The model under review builds one solid part; all positions refer to its coordinate system, in mm. Coordinates: 2 decimals unless noted, no trailing zeros. Loops run counter-clockwise (first coordinate to the right, second up) from the corner with the lowest first, then second, coordinate; pieces in that order, holes last. Notation, with made-up numbers: M 56,-20 L 82,-20 A29 ccw 82,4 Z; hole C 27.5,53 d3. An arc over 180 degrees is marked long. Write item = value, one per line. Start each with the question number.
Q1. We need section A-A on y = -17. Give the boundary of the cut face in (x, z), and give its area (3 significant figures).
Q2. We need section B-B on z = 1.65. Give the boundary of the cut face in (x, y).
Q3. Wall thickness on probe 1 along X at (y, z) = (-13, 4.15); probe 2 along Y at (x, z) = (139, 0.3); probe 3 along X at (y, z) = (6.5, 2.55): over which ranges is each line inside the solid? List them lowest first.
Q4. Clearance check with flat-ended pins moving along their axes: pin 1 Ø2.5 at (x, z) = (-83, 3.5) entering from -Y; pin 2 Ø1.5 at (y, z) = (13.5, 3.5) entering from -X; pin 3 Ø2.5 at (y, z) = (18, 1.5) entering from +X. State where each tip first meets the part, or that it passes through.
Q5. We need section C-C on x = 144.5. Give the boundary of the cut face in (y, z).
from build123d import *

# Parameters (mm, degrees)
BOSS_EXTRUDE1_DEPTH     = 5
ESQUISSE1_W             = 320
ESQUISSE1_H             = 50
ENL_V_MAT_EXTRU_1_DEPTH = 10
CONG_1_R                = 5


with BuildPart() as part:
    # Sketch1 → Boss-Extrude1 (new body)
    with BuildSketch(Plane.XY):
        Polygon((-75.813253012, 35), (254.186746988, 35), (254.186746988, 17.5), (254.186746988, 7.5), (264.186746988, 7.5), (264.186746988, -7.5), (254.186746988, -7.5), (254.186746988, -17.5), (254.186746988, -35), (-75.813253012, -35), (-75.813253012, -17.5), (-75.813253012, -7.5), (-85.813253012, -7.5), (-85.813253012, 7.5), (-75.813253012, 7.5), (-75.813253012, 17.5), align=None)
    extrude(amount=BOSS_EXTRUDE1_DEPTH)

    # Esquisse1 → Enlèv. mat.-Extru.1 (cut)
    with BuildSketch(Plane.XY.offset(5)):
        with Locations((89.186746988, 0)):
            Rectangle(ESQUISSE1_W, ESQUISSE1_H)
    extrude(amount=-ENL_V_MAT_EXTRU_1_DEPTH, mode=Mode.SUBTRACT)

    # Congé1
    cong_1_edges = [part.edges().sort_by_distance(p)[0] for p in [
        (-75.813253012, 35, 2.5),
        (254.186746988, 35, 2.5),
        (254.186746988, -35, 2.5),
        (-75.813253012, -35, 2.5),
        (-70.813253012, -25, 2.5),
        (-70.813253012, 25, 2.5),
        (249.186746988, 25, 2.5),
        (249.186746988, -25, 2.5),
    ]]
    fillet(cong_1_edges, radius=CONG_1_R)


solid = part.part
Returned:
q1.outline = M -75.81,0 L -70.81,0 L -70.81,5 L -75.81,5 Z; M 249.19,0 L 254.19,0 L 254.19,5 L 249.19,5 Z
q1.area = 50.0 mm^2
q2.outline = M -85.81,-7.5 L -75.81,-7.5 L -75.81,-30 A5 ccw -70.81,-35 L 249.19,-35 A5 ccw 254.19,-30 L 254.19,-7.5 L 264.19,-7.5 L 264.19,7.5 L 254.19,7.5 L 254.19,30 A5 ccw 249.19,35 L -70.81,35 A5 ccw -75.81,30 L -75.81,7.5 L -85.81,7.5 Z; hole M -70.81,-20 A5 ccw -65.81,-25 L 244.19,-25 A5 ccw 249.19,-20 L 249.19,20 A5 ccw 244.19,25 L -65.81,25 A5 ccw -70.81,20 Z
q3.probe_1 = -75.81 to -70.81, 249.19 to 254.19
q3.probe_2 = -35 to -25, 25 to 35
q3.probe_3 = -85.81 to -70.81, 249.19 to 264.19
q4.pin_1 = -7.5
q4.pin_2 = -75.81
q4.pin_3 = 254.19
q5.outline = M -35,0 L -25,0 L -25,5 L -35,5 Z; M 25,0 L 35,0 L 35,5 L 25,5 Z
